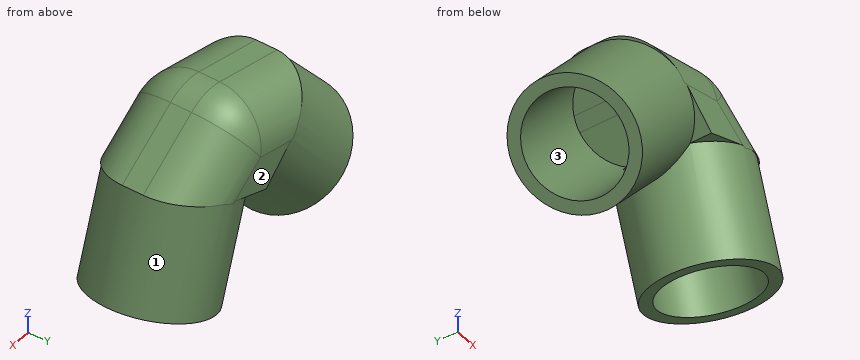
from build123d import *

# Parameters (mm, degrees)
F2_R          = 14.2875
F2_R_2        = 11.43
F5_R          = 14.2875
F5_R_2        = 11.43
F7_DEPTH      = 14.2875
F7_DEPTH_BACK = 14.2875
F8_T1_DEPTH   = 48.1632201407
F8_T3_DEPTH   = 48.1632201407
F8_T5_DEPTH   = 5.08
F8_T10_DEPTH  = 11.7475
F8_T16_DEPTH  = 11.7475


# Not quite as in the source:
# - a fillet or chamfer that OpenCascade refuses, or shapes differently, is made with other operations: its cross-section is extruded or revolved along the edge and cut away or added


with BuildPart() as f3:
    # F3: sweep along a path in F0
    with BuildLine(Plane.XZ) as f3_path:
        Line((43.6000298417, -8.651005595), (35.4240159518, 15.3971294028))
    # F2 (on line) → F3 (sweep)
    with BuildSketch(Plane(origin=(7.1540121537, 0, -21.0421181231), x_dir=(0.9467769684, 0, 0.3218903106), z_dir=(-0.3218903106, 0, 0.9467769684))):
        with Locations((38.471757228, 0)):
            Circle(F2_R)
        with Locations((38.471757228, 0)):
            Circle(F2_R_2, mode=Mode.SUBTRACT)
    sweep(path=f3_path.line)

    # F6: sweep along a path in F0
    with BuildLine(Plane.XZ) as f6_path:
        Line((0, 0), (16.7382888768, 19.1047032292))
    # F5 (on face) → F6 (sweep)
    with BuildSketch(Plane(origin=(0, 0, 0), x_dir=(0.7521536704, 0, -0.6589877511), z_dir=(0.6589877511, 0, 0.7521536704))):
        Circle(F5_R)
        Circle(F5_R_2, mode=Mode.SUBTRACT)
    sweep(path=f6_path.line)

    # F0 (on Front) → F7 (join, two sides)
    with BuildSketch(Plane.XZ) as f7_sk:
        with BuildLine():
            Line((14.1742345569, 21.3511595802), (16.7382888768, 19.1047032292))
            Line((16.7382888768, 19.1047032292), (29.2920055344, 33.4332306512))
            Line((29.2920055344, 33.4332306512), (25.1637988833, 32.5627254125))
            add(Edge.make_bspline(
                [(14.1742345569, 21.3511595802), (18.1555587274, 26.691715757), (21.8910272526, 30.7931889907), (25.1637988833, 32.5627254125)],
                knots=[0.2192972469, 0.2192972469, 0.2192972469, 0.2192972469, 0.4127143591, 0.4127143591, 0.4127143591, 0.4127143591], degree=3))
        make_face()
        Polygon((29.2920055344, 33.4332306512), (16.7382888768, 19.1047032292), (25.0025134025, 11.8539710829), (25.0108680409, 11.8568115377), align=None)
        with BuildLine():
            Line((5.9918933103, 28.5199907224), (14.1742345569, 21.3511595802))
            add(Edge.make_bspline(
                [(14.1742345569, 21.3511595802), (18.1555587274, 26.691715757), (21.8910272526, 30.7931889907), (25.1637988833, 32.5627254125)],
                knots=[0.2192972469, 0.2192972469, 0.2192972469, 0.2192972469, 0.4127143591, 0.4127143591, 0.4127143591, 0.4127143591], degree=3))
            Line((25.1637988833, 32.5627254125), (5.9918933103, 28.5199907224))
        make_face()
        with BuildLine():
            Line((32.7751119786, 31.0525082771), (29.2920055344, 33.4332306512))
            Line((29.2920055344, 33.4332306512), (35.4240159518, 15.3971294028))
            Line((35.4240159518, 15.3971294028), (38.6515313802, 16.4944374051))
            add(Edge.make_bspline(
                [(32.7751119786, 31.0525082771), (35.1243349239, 28.1674701754), (37.0108609747, 22.9504952618), (38.6515313802, 16.4944374051)],
                knots=[0.5872856409, 0.5872856409, 0.5872856409, 0.5872856409, 0.7807027531, 0.7807027531, 0.7807027531, 0.7807027531], degree=3))
        make_face()
        Polygon((35.4240159518, 15.3971294028), (29.2920055344, 33.4332306512), (25.0108680409, 11.8568115377), align=None)
        with BuildLine():
            Line((48.951091888, 19.9961372159), (32.7751119786, 31.0525082771))
            add(Edge.make_bspline(
                [(32.7751119786, 31.0525082771), (35.1243349239, 28.1674701754), (37.0108609747, 22.9504952618), (38.6515313802, 16.4944374051)],
                knots=[0.5872856409, 0.5872856409, 0.5872856409, 0.5872856409, 0.7807027531, 0.7807027531, 0.7807027531, 0.7807027531], degree=3))
            Line((38.6515313802, 16.4944374051), (48.951091888, 19.9961372159))
        make_face()
    extrude(amount=F7_DEPTH)
    extrude(f7_sk.sketch, amount=-F7_DEPTH_BACK)

    # F8: fillet of radius 11.7475 on 5 edges, made by hand

    # F8_s2 → F8_t1 (cut)
    with BuildSketch(Plane(origin=(48.2948087603, 0, -33.0097668872), x_dir=(0, 1, 0), z_dir=(-0.8255784296, 0, 0.5642873884))):
        with BuildLine():
            ThreePointArc((14.2875, -32.3833633586), (10.846736912, -40.6901002706), (2.54, -44.1308633586))
            Line((2.54, -44.1308633586), (14.2875, -44.1308633586))
            Line((14.2875, -44.1308633586), (14.2875, -32.3833633586))
        make_face()
        with BuildLine():
            ThreePointArc((-2.54, -44.1308633586), (-10.846736912, -40.6901002706), (-14.2875, -32.3833633586))
            Line((-14.2875, -32.3833633586), (-14.2875, -44.1308633586))
            Line((-14.2875, -44.1308633586), (-2.54, -44.1308633586))
        make_face()
    extrude(amount=F8_T1_DEPTH, mode=Mode.SUBTRACT)

    # F8_s4 → F8_t3 (cut)
    with BuildSketch(Plane(origin=(29.884780339, 0, 6.3017334256), x_dir=(0, 1, 0), z_dir=(-0.9784824031, 0, -0.2063302857))):
        with BuildLine():
            ThreePointArc((14.2875, -14.9225), (10.846736912, -23.229236912), (2.54, -26.67))
            Line((2.54, -26.67), (14.2875, -26.67))
            Line((14.2875, -26.67), (14.2875, -14.9225))
        make_face()
        with BuildLine():
            ThreePointArc((-14.2875, -14.9225), (-10.846736912, -23.229236912), (-2.54, -26.67))
            Line((-2.54, -26.67), (-14.2875, -26.67))
            Line((-14.2875, -26.67), (-14.2875, -14.9225))
        make_face()
    extrude(amount=F8_T3_DEPTH, mode=Mode.SUBTRACT)

    # F8_s6 → F8_t5 (cut)
    with BuildSketch(Plane.XZ.offset(-2.54)):
        with BuildLine():
            ThreePointArc((33.434782745, 30.6016196872), (29.0921538432, 32.4260021156), (24.3819516188, 32.3978591166))
            Line((24.3819516188, 32.3978591166), (29.2920055344, 33.4332306512))
            Line((29.2920055344, 33.4332306512), (33.434782745, 30.6016196872))
        make_face()
    extrude(amount=F8_T5_DEPTH, mode=Mode.SUBTRACT)


with BuildPart() as f8_tool8:
    # F8_s9 → F8_t10 (new body)
    with BuildSketch(Plane.XZ.offset(-2.54)):
        Polygon((26.8058166503, 20.903137086), (33.434782745, 30.6016196872), (29.2920055344, 33.4332306512), (24.3819516188, 32.3978591166), align=None)
    extrude(amount=-F8_T10_DEPTH)

    # F8_s11 → F8_t12 (revolve, cut)
    with BuildSketch(Plane(origin=(26.8058166503, 2.54, 20.903137086), x_dir=(-0.194623298, 0, -0.9808780617), z_dir=(0.9808780617, 0, -0.194623298))):
        with BuildLine():
            ThreePointArc((0, -11.7475), (11.7475, 0), (0, 11.7475))
            Line((0, 11.7475), (0, -11.7475))
        make_face()
    revolve(axis=Axis((26.8058166503, 2.54, 20.903137086), (0, 1, 0)), mode=Mode.SUBTRACT)


with BuildPart() as f3_1:
    add(f3.part)

    # F8_t7: cut F8_tool8
    add(f8_tool8.part, mode=Mode.SUBTRACT)


with BuildPart() as f8_tool14:
    # F8_s15 → F8_t16 (new body)
    with BuildSketch(Plane.XZ.offset(2.54)):
        Polygon((26.8058166503, 20.903137086), (24.3819516188, 32.3978591166), (29.2920055344, 33.4332306512), (33.434782745, 30.6016196872), align=None)
    extrude(amount=F8_T16_DEPTH)

    # F8_s17 → F8_t18 (revolve, cut)
    with BuildSketch(Plane(origin=(26.8058166503, -2.54, 20.903137086), x_dir=(-0.194623298, 0, -0.9808780617), z_dir=(-0.9808780617, 0, 0.194623298))):
        with BuildLine():
            ThreePointArc((0, -11.7475), (11.7475, 0), (0, 11.7475))
            Line((0, 11.7475), (0, -11.7475))
        make_face()
    revolve(axis=Axis((26.8058166503, -2.54, 20.903137086), (0, -1, 0)), mode=Mode.SUBTRACT)


with BuildPart() as f3_2:
    add(f3_1.part)

    # F8_t13: cut F8_tool14
    add(f8_tool14.part, mode=Mode.SUBTRACT)


solid = f3_2.part
Design review of the part built by this model. Coordinates are the model's own, in mm. Face numbers are marked on the shaded views. Give positions to 0.01 mm unless a question says otherwise; leave off trailing zeros. Order: outer loops, then holes, each group sorted by start corner. A loop starts at its lowest first (then second) coordinate and runs counter-clockwise, first axis right, second up. Notation, with made-up numbers: (27.25, -6) - (72.25, -6) arc R8 cw to (72.25, 7) - close; hole circle Ø6 at (78, 18.5). An arc over 180 degrees is marked (long way). Use CSV: the item, a comma, the result in double quotes. Start each with the question number.
Q1. For line 1 (Y direction, x = 45.5, z = -3.5); line 2 (X direction, y = -5.5, z = 7); line 3 (X direction, y = 6.5, z = 3.5), list the stretches that pass through material, from the lowest coordinate up.
Q2. Take a section at B-B (z = 4). Count the separate pieces of the cut face and the enclosed holes in it, and give its area (3 significant figures).
Q3. Take a section at C-C (y = -7.75). State the section outline as (x, z) points, and give its area (3 significant figures).
Q4. For P1, Ø5, axis at y = -1.5, z = 19.5, coming from the +X side; P2, Ø12, axis at y = -5, z = 20, coming from the +X side; P3, Ø1, axis at x = 28, y = -4.5, coming from the +Z side; P4, Ø2, axis at x = 40.5, z = 27.5, coming from the -Y side, all flat-tipped, find the tip position at first contact; note any pin that passes through.
Q5. Draft analysis for pull direction Y (two halves, no side actions). For the marked faces 1, 2 and 3, state which applies: pulls with the +Y half, pulls with the -Y half, needs draft (parallel to the pull), parting line crosses it, or undercut.
Calculated:
1,line 1,"y = -13.86 to -10.89, 10.89 to 13.86"
1,line 2,"x = -7.99 to -7.19, 19.45 to 23.66, 24.33 to 27.67, 48.84 to 52.18"
1,line 3,"x = 15.57 to 19.98, 26.01 to 29.51, 49.37 to 52.88"
2,separate pieces,"2"
2,enclosed holes,"1"
2,area,"445 mm²"
3,outline,"(-9.03, 7.91) - (-6.32, 5.54) - (10.42, 24.64) - (16.74, 19.1) - (23.05, 13.56) - (6.32, -5.54) - (9.03, -7.91) - (24.6, 9.87) - (32.21, -12.52) - (35.62, -11.36) - (27.45, 12.69) - (43.36, 18.09) - (51.53, -5.95) - (54.94, -4.79) - (46.77, 19.25) - (47.51, 19.51) - (32.75, 29.6) arc R10.53 ccw to (24.63, 31.21) - (7.14, 27.52) - (7.71, 27.01) - close"
3,area,"787 mm²"
4,P1,"stops at x = 49.89"
4,P2,"stops at x = 50.55"
4,P3,"stops at z = 32.51"
4,P4,"passes through"
5,face 1,"parting line crosses it"
5,face 2,"pulls with the +Y half"
5,face 3,"undercut"
